Work out the finished part from the listing and answer in its coordinate system (mm). A direction names the side the tool comes from. Coordinates: 2 decimals unless noted, no trailing zeros. Order: outer loops, then holes, each group sorted by start corner. A loop starts at its lowest first (then second) coordinate and runs counter-clockwise, first axis right, second up. Notation, with made-up numbers: (-13, 17.5) -> (38, 17.5) arc R8 ccw to (38, 26.5) -> close; hole circle Ø5 at (36, 4.25). An arc over 180 degrees is marked (long way). Write item = value, one per line. Start each with the question number.
Q1. Which of the six approach directions +Z, -Z, +X, -X, +Y, -Y give full straight-line access (tool end or side, diameter ignored) to faces 5 (the flat face through (-1, 30, -1)), 6 (the flat face through (-1, 10, -25)), 7 (the flat face through (30, 49, -43)), 8 (the flat face through (50, 40, -15))?
Q2. For a pull along Y with two mould halves and no side action, classify faces 1 (the cylindrical face through (-40.14, 50.357, -48.252)), 2 (the cylindrical face through (39.86, 50.357, -48.252)), 3 (the flat face through (-50, 40, -15)), 4 (the flat face through (-1, 0, -47)) as +Y half, -Y half, draft (parallel to the pull), parting line (faces both ways), or undercut.
Q3. The part is cut by section B-B, the plane z = -45. Determine the outline of the cut face in (x, y).
Q4. The part is cut by section A-A, the plane y = 65. Determine the outline of the cut face in (x, z), plus the area to 3 significant figures.
Q5. The part is cut by section C-C, the plane y = 13. Determine the outline of the cut face in (x, z), plus the area to 3 significant figures.
Q6. Straight lines are drawn through the part: L1, parallel to Z at x = 37, y = 13.5; L2, parallel to X at y = 41.5, z = -9.5; L3, parallel to Y at x = -37, z = -45. For each, find the intervals that lie inside material, in ascending order. Write a range as from..to.
Q7. The part is cut by section D-D, the plane x = 0. Determine the outline of the cut face in (y, z), plus the area to 3 significant figures.
Q8. Flat-ended cylindrical pins translate along their axes: pin 1 (1.5 mm diameter, centred on x = 4.5, z = 21.5, fed in from -Y); pin 2 (6 mm diameter, centred on x = 2.5, z = -46, fed in from +Y). Find the tip coordinate at first contact, or state that the pin passes through.
```python
from build123d import *

# Parameters (mm, degrees)
BOSS_EXTRUDE1_DEPTH      = 50
BOSS_EXTRUDE1_DEPTH_BACK = 50
CUT_EXTRUDE2_DEPTH       = 111.905365064
HOLE1_D                  = 30
SKETCH5_W                = 60
SKETCH5_H                = 70
CUT_EXTRUDE3_DEPTH       = 180.164728672


with BuildPart() as part:
    # Sketch1 → Boss-Extrude1 (new, two sides: drawn at the far end of the back side and taken through both)
    with BuildSketch(Plane(origin=(0, 0, 0), x_dir=(0, 0, -1), z_dir=(1, 0, 0)).offset(-BOSS_EXTRUDE1_DEPTH_BACK)):
        Polygon((-70, 0), (-25, 0), (-25, 20), (25, 20), (25, 0), (70, 0), (70, 100), (30, 100), (0, 30), (-70, 30), align=None)
    extrude(amount=BOSS_EXTRUDE1_DEPTH + BOSS_EXTRUDE1_DEPTH_BACK)

    # Sketch2 → Cut-Extrude2 (cut, through all)
    with BuildSketch(Plane(origin=(0, 30, 0), x_dir=(1, 0, 0), z_dir=(0, 1, 0))):
        with BuildLine():
            Line((-30, -70), (30, -70))
            ThreePointArc((30, -70), (0, -40), (-30, -70))
        make_face()
    extrude(amount=-CUT_EXTRUDE2_DEPTH, mode=Mode.SUBTRACT)

    # Hole1 (through all)
    with Locations(Plane(origin=(50, 0, 0), x_dir=(0, 0, -1), z_dir=(1, 0, 0))):
        with Locations((45, 65)):
            Hole(HOLE1_D / 2)

    # Sketch5 → Cut-Extrude3 (cut, through all)
    with BuildSketch(Plane(origin=(0, 0, -70), x_dir=(-1, 0, 0), z_dir=(0, 0, -1))):
        with Locations((0, 65)):
            Rectangle(SKETCH5_W, SKETCH5_H)
    extrude(amount=-CUT_EXTRUDE3_DEPTH, mode=Mode.SUBTRACT)


solid = part.part
```
Model answer:
q1.face_5 = +Z, +Y
q1.face_6 = +X, -X, -Y
q1.face_7 = +Z, -Z, +Y
q1.face_8 = +Z, -Z, +X, +Y, -Y
q2.face_1 = undercut
q2.face_2 = undercut
q2.face_3 = draft
q2.face_4 = -Y half
q3.outline = (-50, 0) -> (50, 0) -> (50, 50) -> (30, 50) -> (30, 30) -> (-30, 30) -> (-30, 50) -> (-50, 50) -> close; (-50, 80) -> (-30, 80) -> (-30, 100) -> (-50, 100) -> close; (30, 80) -> (50, 80) -> (50, 100) -> (30, 100) -> close
q4.outline = (-50, -70) -> (-30, -70) -> (-30, -60) -> (-50, -60) -> close; (-50, -30) -> (-30, -30) -> (-30, -15) -> (-50, -15) -> close; (30, -70) -> (50, -70) -> (50, -60) -> (30, -60) -> close; (30, -30) -> (50, -30) -> (50, -15) -> (30, -15) -> close
q4.area = 1,000 mm2
q5.outline = (-50, -70) -> (50, -70) -> (50, -25) -> (-50, -25) -> close; (-50, 25) -> (50, 25) -> (50, 70) -> (30, 70) arc R30 cw to (-30, 70) -> (-50, 70) -> close
q5.area = 7,590 mm2
q6.L1 = -70..-25, 25..70
q6.L2 = -50..-30, 30..50
q6.L3 = 0..50, 80..100
q7.outline = (0, -70) -> (30, -70) -> (30, 40) -> (0, 40) -> (0, 25) -> (20, 25) -> (20, -25) -> (0, -25) -> close
q7.area = 2,300 mm2
q8.pin_1 = 20
q8.pin_2 = 30
